```python
from build123d import *

# Parameters (mm, degrees)
F0_R     = 3.175
F1_DEPTH = 6.35
F3_D     = 2.5781
F3_DEPTH = 13.905
F3_TIP   = 0.774539381
F5_D     = 4.5
F6_D     = 4.5
F6_DEPTH = 12
F6_TIP   = 1.3519363928
F7_D     = 4.5
F7_DEPTH = 12
F7_TIP   = 1.3519363928
F8_D     = 2.5


with BuildPart() as f1:
    # F0 (on Top) → F1 (new body)
    with BuildSketch(Plane.XY):
        Polygon((-180, 60), (-120, 0), (120, 0), (180, 60), (180, 220), (120, 280), (-120, 280), (-180, 220), align=None)
        with Locations((0, 20)):
            Circle(F0_R, mode=Mode.SUBTRACT)
        with Locations((-160, 140)):
            Circle(F0_R, mode=Mode.SUBTRACT)
        with Locations((160, 140)):
            Circle(F0_R, mode=Mode.SUBTRACT)
        with Locations((0, 260)):
            Circle(F0_R, mode=Mode.SUBTRACT)
    extrude(amount=F1_DEPTH)

    # F3
    with Locations(Plane.XY.offset(6.35)):
        with Locations((-15.5, 155.5), (15.5, 155.5), (15.5, 124.5), (-15.5, 124.5)):
            Hole(F3_D / 2, depth=F3_DEPTH)
            with Locations((0, 0, -(F3_DEPTH + F3_TIP / 2))):  # 118° drill point
                Cone(0, F3_D / 2, F3_TIP, mode=Mode.SUBTRACT)

    # F5 (through all)
    with Locations(Plane.XY.offset(6.35)):
        with Locations((-160.553125, 167.94), (-160.553125, 112.06), (160.553125, 112.06), (160.553125, 167.94)):
            Hole(F5_D / 2)

    # F6
    with Locations(Plane.XY.offset(6.35)):
        with Locations((-151.2489651369, 221.2489651369), (-121.2489651369, 251.2489651369)):
            Hole(F6_D / 2, depth=F6_DEPTH)
            with Locations((0, 0, -(F6_DEPTH + F6_TIP / 2))):  # 118° drill point
                Cone(0, F6_D / 2, F6_TIP, mode=Mode.SUBTRACT)

    # F7
    with Locations(Plane.XY.offset(6.35)):
        with Locations((121.2489651369, 251.2489651369), (151.2489651369, 221.2489651369), (-151.2489651369, 58.7510348631), (-121.2489651369, 28.7510348631), (121.2489651369, 28.7510348631), (151.2489651369, 58.7510348631)):
            Hole(F7_D / 2, depth=F7_DEPTH)
            with Locations((0, 0, -(F7_DEPTH + F7_TIP / 2))):  # 118° drill point
                Cone(0, F7_D / 2, F7_TIP, mode=Mode.SUBTRACT)

    # F8 (through all)
    with Locations(Plane(origin=(0, 0, 0), x_dir=(1, 0, 0), z_dir=(0, 0, -1))):
        with Locations((-123.65, -148), (-115.65, -140), (-123.65, -132), (-131.65, -140), (123.65, -148), (131.65, -140), (115.65, -140), (123.65, -132)):
            Hole(F8_D / 2)


solid = f1.part
```
Part model, mm, in its own coordinate system. Round coordinates to 2 decimals unless told otherwise and drop trailing zeros.
Item 1: Drill centre lines: line 1 (X direction, y = 124.5, z = 5.25); line 2 (X direction, y = 167.94, z = 3.5); line 3 (Y direction, x = 15.5, z = 2.75). Where is each one in solid material? Low to high.
Item 2: Drop a flat-ended pin along its axis: P1, Ø5.5, axis at x = -160, y = 140, coming from the -Z side. Give the stop position or say it passes through.
Item 3: Cut at A-A, the plane z = 4.5. State how many separate pieces and enclosed holes the cut face has, then the cut area to 3 significant figures.
Item 4: Mould opens along Y. For faces 1 (the face through (-150, 30, 3)), 2 (the face through (150, 250, 3)), 3 (the face through (-3, 142, 0)) say: +Y half, -Y half, draft (parallel to the pull), parting line (faces both ways), or undercut.
A:
1. line 1: x = -180 to -16.79, -14.21 to 14.21, 16.79 to 180
1. line 2: x = -180 to -162.8, -158.3 to 158.3, 162.8 to 180
1. line 3: y = 0 to 123.21, 125.79 to 154.21, 156.79 to 280
2. P1: passes through
3. separate pieces: 1
3. enclosed holes: 28
3. area: 93,200 mm2
4. face 1: -Y half
4. face 2: +Y half
4. face 3: draft
